Can you work these out from the model? Positions are in its coordinate system, mm. A direction names the side the tool comes from. Coordinates: 2 decimals unless noted, no trailing zeros. Write each loop counter-clockwise with the first axis right and the second up, starting at its lowest first coordinate (ties: lowest second). Pieces come first, ordered by that corner, then holes.
Autodesk Inventor part; units mm, degrees
ref_plane "YZ Plane" through (0, 0, 0) normal (1, 0, 0) x (0, 1, 0)
ref_plane "XZ Plane" through (0, 0, 0) normal (0, 1, 0) x (-1, 0, 0)
ref_plane "XY Plane" through (0, 0, 0) normal (0, 0, 1) x (1, 0, 0)
sketch "Náčrt1" plane through (0, 0, 0) normal (0, 0, 1) x (1, 0, 0)
  line L0 (0, 0) -> (7.6, 0)
  line L1 (7.6, 0) -> (7.6, 2.6)
  line L2 (7.6, 2.6) -> (0, 2.6)
  line L3 (0, 2.6) -> (0, 0)
  dimension "d0" = 7.6
  dimension "d1" = 2.6
extrude "Vysunutí1" add sketch "Náčrt1" along normal blind 2.5
chamfer "Zkosení1" distance 0.9 angle 60 1 edges at (0, 2.6, 1.25) measured on face at (0, 1.7333, 0.8333)
chamfer "Zkosení2" distance 0.9 angle 60 1 edges at (7.6, 2.6, 1.25) measured on face at (7.6, 0.8667, 0.8333)
sketch "Náčrt2" plane through (0, 0, 2.5) normal (0, 0, 1) x (1, 0, 0)
  line L0 (-1.2, -0.7) -> (8.8, -0.7)
  line L1 (8.8, -0.7) -> (8.8, 3.3)
  line L2 (8.8, 3.3) -> (-1.2, 3.3)
  line L3 (-1.2, 3.3) -> (-1.2, -0.7)
  line L4 (-1.2, -0.7) -> (8.8, 3.3) construction
  line L5 (8.8, -0.7) -> (-1.2, 3.3) construction
  line L6 (0, 0) -> (7.6, 0)
  point P0 (3.8, 1.3)
  dimension "d10" = 10
  dimension "d11" = 4
  dimension "d12" = 1.3
extrude "Vysunutí2" add sketch "Náčrt2" along normal blind 1
properties part number "ChargeCover"
1. I'm going to push flat-ended pins straight in: P1, Ø0.8, axis at x = 4, z = 1, coming from the -Y side; P2, Ø0.8, axis at y = 0.5, z = 1.5, coming from the -X side; P3, Ø0.5, axis at y = 1, z = 1, coming from the +X side. Where does each tip first touch, or does it pass through?
2. If we section it at C-C, the plane x = 5.5: List the corners of the cut face in (y, z) for me, plus the area to 3 significant figures.
3. If we section it at A-A, the plane y = 0.9: List the corners of the cut face in (x, z) for me, plus the area to 3 significant figures.
4. If we section it at B-B, the plane z = 0.75: List the corners of the cut face in (x, y) for me.
5. Which directions (+Z, -Z, +X, -X, +Y, -Y) give clear straight access to the entire face, cutting with the end or side of a thin tool? Please do faces 1 (the face through (4, 0, 1)), 2 (the face through (6.81, 2.156, 1.267)), 3 (the face through (4, 2.6, 1)).
6. If we section it at D-D, the plane y = -0.1: List the corners of the cut face in (x, z) for me, plus the area to 3 significant figures.
7. If I drill on L1, parallel to Z at x = 8, y = 0.25; L2, parallel to Y at x = 2, z = 0.2; L3, parallel to X at y = 1.4, z = 1.8, over which ranges is the centre line in solid material (lowest first)?
Answers:
1. P1: stops at y = 0
1. P2: stops at x = 0
1. P3: stops at x = 7.6
2. outline: (-0.7, 2.5) - (0, 2.5) - (0, 0) - (2.6, 0) - (2.6, 2.5) - (3.3, 2.5) - (3.3, 3.5) - (-0.7, 3.5) - close
2. area: 10.5 mm2
3. outline: (-1.2, 2.5) - (0, 2.5) - (0, 0) - (7.6, 0) - (7.6, 2.5) - (8.8, 2.5) - (8.8, 3.5) - (-1.2, 3.5) - close
3. area: 29.0 mm2
4. outline: (0, 0) - (7.6, 0) - (7.6, 1.7) - (6.04, 2.6) - (1.56, 2.6) - (0, 1.7) - close
5. face 1: -Z, +X, -X, -Y
5. face 2: -Z, +X, +Y
5. face 3: -Z, +X, -X, +Y
6. outline: (-1.2, 2.5) - (8.8, 2.5) - (8.8, 3.5) - (-1.2, 3.5) - close
6. area: 10.0 mm2
7. L1: z = 2.5 to 3.5
7. L2: y = 0 to 2.6
7. L3: x = 0 to 7.6
